For this review, take the finished solid that the model builds, in its own axes (mm). A direction names the side the tool comes from. Round coordinates to 2 decimals unless told otherwise and drop trailing zeros. Write each loop counter-clockwise with the first axis right and the second up, starting at its lowest first coordinate (ties: lowest second). Pieces come first, ordered by that corner, then holes.
from build123d import *

# Parameters (mm, degrees)
F1_DEPTH = 19.05
F2_W     = 101.6
F2_H     = 19.05
F3_DEPTH = 19.05


with BuildPart() as f1:
    # F0 (on Front) → F1 (new body)
    with BuildSketch(Plane.XZ):
        Polygon((304.8, 660.4), (51.1001483644, 660.4), (58.9155329798, 558.8), (312.6153846154, 558.8), align=None)
        Polygon((94.084763749, 101.6), (101.9001483644, 0), (355.6, 0), (347.7846153846, 101.6), align=None)
        Polygon((-238.0690824048, 203.2), (-245.8844670202, 101.6), (-7.8153846154, 101.6), (-15.6307692308, 203.2), align=None)
        Polygon((326.2923076923, 381), (72.5924560567, 381), (80.4078406721, 279.4), (334.1076923077, 279.4), align=None)
        Polygon((-202.8998516356, 660.4), (-304.8, 660.4), (-355.6, 0), (-253.6998516356, 0), (-245.8844670202, 101.6), (-238.0690824048, 203.2), (-210.715236251, 558.8), align=None)
        Polygon((51.1001483644, 660.4), (-50.8, 660.4), (-42.9846153846, 558.8), (-15.6307692308, 203.2), (-7.8153846154, 101.6), (0, 0), (101.9001483644, 0), (94.084763749, 101.6), (80.4078406721, 279.4), (72.5924560567, 381), (58.9155329798, 558.8), align=None)
        Polygon((-50.8, 660.4), (-202.8998516356, 660.4), (-210.715236251, 558.8), (-42.9846153846, 558.8), align=None)
    extrude(amount=F1_DEPTH)

    # F2 (on face) → F3 (join, through all)
    with BuildSketch(Plane.XZ.offset(19.05)):
        with Locations((203.2, 669.925)):
            Rectangle(F2_W, F2_H)
        with Locations((-203.2, 669.925)):
            Rectangle(F2_W, F2_H)
    extrude(amount=-F3_DEPTH)


solid = f1.part
(1) For line 1 along Z through (x, y) = (225, -8.5); line 2 along Z through (x, y) = (102, -9.25); line 3 along Z through (x, y) = (-113.5, -9.5), list the stretches that pass through material, from the lowest coordinate up.
Geometry check:
line 1: z = 0 to 101.6, 279.4 to 381, 558.8 to 679.45
line 2: z = 0 to 101.6, 279.4 to 381, 558.8 to 660.4
line 3: z = 101.6 to 203.2, 558.8 to 660.4
(2) We need section A-A, the plane x = 279.5. Give the boundary of the cut face in (y, z).
Geometry check:
outline: (-19.05, 0) - (0, 0) - (0, 101.6) - (-19.05, 101.6) - close; (-19.05, 279.4) - (0, 279.4) - (0, 381) - (-19.05, 381) - close; (-19.05, 558.8) - (0, 558.8) - (0, 660.4) - (-19.05, 660.4) - close
(3) For faces 5 (the face through (-4, -9, 52)), 6 (the face through (254, -10, 670)), 7 (the face through (2, -9, 660.4)), 8 (the face through (-254, -10, 670)), 9 (the face through (201, -9, 381)), list the 3-axis set-ups (+Z, -Z, +X, -X, +Y, -Y) from which the entire face can be reached by the end or side of a thin tool; tool diameter is ignored.
Geometry check:
face 5: -Z, +Y, -Y
face 6: +Z, +X, +Y, -Y
face 7: +Z, +Y, -Y
face 8: +Z, -X, +Y, -Y
face 9: +X, +Y, -Y
(4) We need section C-C, the plane z = 254. Give the boundary of the cut face in (x, y), and give its area (3 significant figures).
Geometry check:
outline: (-336.06, -19.05) - (-234.16, -19.05) - (-234.16, 0) - (-336.06, 0) - close; (-19.54, -19.05) - (82.36, -19.05) - (82.36, 0) - (-19.54, 0) - close
area: 3,880 mm2
(5) For pin 1 Ø5.5 at (y, z) = (-7, 671.5) entering from -X; pin 2 Ø6 at (y, z) = (-9, 106.5) entering from +X; pin 3 Ø4 at (y, z) = (-15.5, 483) entering from +X, all flat-tipped, find the tip position at first contact; note any pin that passes through.
Geometry check:
pin 1: stops at x = -254
pin 2: stops at x = 93.94
pin 3: stops at x = 64.9
(6) We need section B-B, the plane y = -6. Give the boundary of the cut face in (x, z).
Geometry check:
outline: (-355.6, 0) - (-253.7, 0) - (-245.88, 101.6) - (-7.82, 101.6) - (0, 0) - (355.6, 0) - (347.78, 101.6) - (94.08, 101.6) - (80.41, 279.4) - (334.11, 279.4) - (326.29, 381) - (72.59, 381) - (58.92, 558.8) - (312.62, 558.8) - (304.8, 660.4) - (254, 660.4) - (254, 679.45) - (152.4, 679.45) - (152.4, 660.4) - (-152.4, 660.4) - (-152.4, 679.45) - (-254, 679.45) - (-254, 660.4) - (-304.8, 660.4) - close; hole (-238.07, 203.2) - (-15.63, 203.2) - (-42.98, 558.8) - (-210.72, 558.8) - close
(7) Mouldability with a two-part tool opening along X and no side actions: class faces 1 (the face through (65.85, -9.39, 468.66)), 2 (the face through (175, -9, 0)), 3 (the face through (-224.584, -9.392, 378.511)), 4 (the face through (-128, -9, 558.8)) as pulls with the +X half, pulls with the -X half, needs draft (parallel to the pull), parting line crosses it, or undercut.
Geometry check:
face 1: pulls with the +X half
face 2: needs draft
face 3: undercut
face 4: undercut
(8) We need section D-D, the plane x = 28.5. Give the boundary of the cut face in (y, z).
Geometry check:
outline: (-19.05, 0) - (0, 0) - (0, 660.4) - (-19.05, 660.4) - close
